Geometry: final body of the model. Coordinates: model frame, mm. A direction names the side the tool comes from. Round coordinates to 2 decimals unless told otherwise and drop trailing zeros. Loops run counter-clockwise (first coordinate to the right, second up) from the corner with the lowest first, then second, coordinate; pieces in that order, holes last. Notation, with made-up numbers: (14, 40) - (24, 40) arc R20 ccw to (24, 76) - close; hole circle Ø3 at (14.5, -38.75). An arc over 180 degrees is marked (long way). Answer in a Markdown table with one row per item. Add a question column.
from build123d import *

# Parameters (mm, degrees)
SKETCH1_R           = 5.5
BOSS_EXTRUDE2_DEPTH = 8.5
SKETCH3_W           = 3.2
SKETCH3_H           = 5.5
CUT_EXTRUDE1_DEPTH  = 6
BOSS_EXTRUDE3_DEPTH = 8.5


with BuildPart() as part:
    # Sketch1 → Boss-Extrude2 (new body)
    with BuildSketch(Plane.XY.offset(20)):
        with Locations((0, 20.92523633)):
            Circle(SKETCH1_R)
    extrude(amount=BOSS_EXTRUDE2_DEPTH)

    # Sketch3 → Cut-Extrude1 (cut)
    with BuildSketch(Plane.XY.offset(28.5)):
        with Locations((0, 20.92523633)):
            Rectangle(SKETCH3_W, SKETCH3_H)
    extrude(amount=-CUT_EXTRUDE1_DEPTH, mode=Mode.SUBTRACT)

    # Sketch4 → Boss-Extrude3 (add)
    with BuildSketch(Plane.XY.offset(20)):
        with BuildLine():
            Line((-0.612805484, 27.420090848), (-0.683508693, 26.382599784))
            ThreePointArc((-0.683508693, 26.382599784), (0, 26.42523633), (0.683508693, 26.382599784))
            Line((0.683508693, 26.382599784), (0.612805484, 27.420090848))
            ThreePointArc((0.612805484, 27.420090848), (0.791416866, 28.376215286), (0.108813843, 29.069128758))
            ThreePointArc((0.108813843, 29.069128758), (0, 29.072382819), (-0.108813843, 29.069128758))
            ThreePointArc((-0.108813843, 29.069128758), (-0.791416866, 28.376215286), (-0.612805484, 27.420090848))
        make_face()
        with BuildLine():
            Line((4.313349752, 25.819485985), (3.760727903, 24.938579779))
            ThreePointArc((3.760727903, 24.938579779), (3.232818888, 25.374829799), (2.654787606, 25.742092438))
            Line((2.654787606, 25.742092438), (3.32180965, 26.539882037))
            ThreePointArc((3.32180965, 26.539882037), (3.739305851, 27.418388093), (4.698827617, 27.577742877))
            ThreePointArc((4.698827617, 27.577742877), (4.788772554, 27.516416295), (4.874892114, 27.449824532))
            ThreePointArc((4.874892114, 27.449824532), (5.01984524, 26.488021768), (4.313349752, 25.819485985))
        make_face()
        with BuildLine():
            Line((6.36634102, 22.349444103), (5.401476877, 21.961598985))
            ThreePointArc((5.401476877, 21.961598985), (5.23081084, 22.624829799), (4.979045272, 23.261709779))
            Line((4.979045272, 23.261709779), (5.987606403, 23.515069401))
            ThreePointArc((5.987606403, 23.515069401), (6.841740827, 23.98039762), (7.711676635, 23.545325605))
            ThreePointArc((7.711676635, 23.545325605), (7.748396757, 23.442843051), (7.778927288, 23.338349376))
            ThreePointArc((7.778927288, 23.338349376), (7.33086335, 22.475033284), (6.36634102, 22.349444103))
        make_face()
        with BuildLine():
            Line((5.987606403, 18.335403259), (4.979045272, 18.588762882))
            ThreePointArc((4.979045272, 18.588762882), (5.23081084, 19.225642861), (5.401476877, 19.888873675))
            Line((5.401476877, 19.888873675), (6.36634102, 19.501028557))
            ThreePointArc((6.36634102, 19.501028557), (7.33086335, 19.375439376), (7.778927288, 18.512123284))
            ThreePointArc((7.778927288, 18.512123284), (7.748396757, 18.407629609), (7.711676635, 18.305147055))
            ThreePointArc((7.711676635, 18.305147055), (6.841740827, 17.87007504), (5.987606403, 18.335403259))
        make_face()
        with BuildLine():
            Line((3.32180965, 15.310590623), (2.654787606, 16.108380222))
            ThreePointArc((2.654787606, 16.108380222), (3.232818888, 16.475642861), (3.760727903, 16.911892881))
            Line((3.760727903, 16.911892881), (4.313349752, 16.030986675))
            ThreePointArc((4.313349752, 16.030986675), (5.01984524, 15.362450892), (4.874892114, 14.400648128))
            ThreePointArc((4.874892114, 14.400648128), (4.788772554, 14.334056365), (4.698827617, 14.272729783))
            ThreePointArc((4.698827617, 14.272729783), (3.739305851, 14.432084567), (3.32180965, 15.310590623))
        make_face()
        with BuildLine():
            Line((-0.612805484, 14.430381812), (-0.683508693, 15.467872876))
            ThreePointArc((-0.683508693, 15.467872876), (0, 15.42523633), (0.683508693, 15.467872876))
            Line((0.683508693, 15.467872876), (0.612805484, 14.430381812))
            ThreePointArc((0.612805484, 14.430381812), (0.791416866, 13.474257374), (0.108813843, 12.781343902))
            ThreePointArc((0.108813843, 12.781343902), (0, 12.778089841), (-0.108813843, 12.781343902))
            ThreePointArc((-0.108813843, 12.781343902), (-0.791416866, 13.474257374), (-0.612805484, 14.430381812))
        make_face()
        with BuildLine():
            Line((-4.313349752, 16.030986675), (-3.760727903, 16.911892881))
            ThreePointArc((-3.760727903, 16.911892881), (-3.232818888, 16.475642861), (-2.654787606, 16.108380222))
            Line((-2.654787606, 16.108380222), (-3.32180965, 15.310590623))
            ThreePointArc((-3.32180965, 15.310590623), (-3.739305851, 14.432084567), (-4.698827617, 14.272729783))
            ThreePointArc((-4.698827617, 14.272729783), (-4.788772554, 14.334056365), (-4.874892114, 14.400648128))
            ThreePointArc((-4.874892114, 14.400648128), (-5.01984524, 15.362450892), (-4.313349752, 16.030986675))
        make_face()
        with BuildLine():
            Line((-6.36634102, 19.501028557), (-5.401476877, 19.888873675))
            ThreePointArc((-5.401476877, 19.888873675), (-5.23081084, 19.225642861), (-4.979045272, 18.588762882))
            Line((-4.979045272, 18.588762882), (-5.987606403, 18.335403259))
            ThreePointArc((-5.987606403, 18.335403259), (-6.841740827, 17.87007504), (-7.711676635, 18.305147055))
            ThreePointArc((-7.711676635, 18.305147055), (-7.748396757, 18.407629609), (-7.778927288, 18.512123284))
            ThreePointArc((-7.778927288, 18.512123284), (-7.33086335, 19.375439376), (-6.36634102, 19.501028557))
        make_face()
        with BuildLine():
            Line((-5.987606403, 23.515069401), (-4.979045272, 23.261709779))
            ThreePointArc((-4.979045272, 23.261709779), (-5.23081084, 22.624829799), (-5.401476877, 21.961598985))
            Line((-5.401476877, 21.961598985), (-6.36634102, 22.349444103))
            ThreePointArc((-6.36634102, 22.349444103), (-7.33086335, 22.475033284), (-7.778927288, 23.338349376))
            ThreePointArc((-7.778927288, 23.338349376), (-7.748396757, 23.442843051), (-7.711676635, 23.545325605))
            ThreePointArc((-7.711676635, 23.545325605), (-6.841740827, 23.98039762), (-5.987606403, 23.515069401))
        make_face()
        with BuildLine():
            Line((-3.32180965, 26.539882037), (-2.654787606, 25.742092438))
            ThreePointArc((-2.654787606, 25.742092438), (-3.232818888, 25.374829799), (-3.760727903, 24.938579779))
            Line((-3.760727903, 24.938579779), (-4.313349752, 25.819485985))
            ThreePointArc((-4.313349752, 25.819485985), (-5.01984524, 26.488021768), (-4.874892114, 27.449824532))
            ThreePointArc((-4.874892114, 27.449824532), (-4.788772554, 27.516416295), (-4.698827617, 27.577742877))
            ThreePointArc((-4.698827617, 27.577742877), (-3.739305851, 27.418388093), (-3.32180965, 26.539882037))
        make_face()
    extrude(amount=BOSS_EXTRUDE3_DEPTH)


solid = part.part
1) Section A-A, the plane x = 5.75. Return the cut outline in (y, z), and give its area (3 significant figures).
2) Reachability of faces 5 (the flat face through (-0.648, 26.909, 24.19)), 6 (the flat face through (1.6, 21, 26)) from +Z, -Z, +X, -X, +Y, -Y: full face, straight path, thin tool, end or side. Return the list, or none.
3) Section C-C, the plane x = -3. Return the cut outline in (y, z).
4) Section B-B, the plane y = 21.5. Return the cut outline in (x, z), and give its area (3 significant figures).
5) Pull-direction query (X, two-part tool) for faces 1 (the flat face through (-2, 21, 28.5)), 2 (the flat face through (4.041, 25.385, 24.19)), 3 (the flat face through (5.49, 18.46, 24.19)), 4 (the cylindrical face through (-5.015, 26.475, 24.19)); classes: pulls with the +X half, pulls with the -X half, needs draft (parallel to the pull), parting line crosses it, or undercut.
6) Contact query for flat-ended pins moving along their axis: pin 1 Ø2 at (y, z) = (26.5, 27.5) entering from -X; pin 2 Ø1 at (x, y) = (-0.5, 21) entering from +Z; pin 3 Ø3 at (x, z) = (5, 25) entering from +Y. Output: stop coordinate, or through.
7) Material intervals for line 1 along X through (y, z) = (15, 25.25); line 2 along X through (y, z) = (23.75, 24.5); line 3 along X through (y, z) = (13.75, 26.5), sorted ascending. Write a range as from..to.
8) Section D-D, the plane y = 17.5. Return the cut outline in (x, z).
Evaluation:
| question | item | result |
|---|---|---|
| 1 | outline | (18.4, 20) - (19.75, 20) - (19.75, 28.5) - (18.4, 28.5) - close; (22.1, 20) - (23.46, 20) - (23.46, 28.5) - (22.1, 28.5) - close |
| 1 | area | 23.0 mm² |
| 2 | face 5 | +Z, -Z |
| 2 | face 6 | +Z |
| 3 | outline | (15.7, 20) - (26.15, 20) - (26.15, 28.5) - (15.7, 28.5) - close |
| 4 | outline | (-5.47, 20) - (5.47, 20) - (5.47, 28.5) - (1.6, 28.5) - (1.6, 22.5) - (-1.6, 22.5) - (-1.6, 28.5) - (-5.47, 28.5) - close |
| 4 | area | 73.8 mm² |
| 5 | face 1 | needs draft |
| 5 | face 2 | pulls with the +X half |
| 5 | face 3 | undercut |
| 5 | face 4 | pulls with the -X half |
| 6 | pin 1 | stops at x = -5.08 |
| 6 | pin 2 | stops at z = 22.5 |
| 6 | pin 3 | stops at y = 27.63 |
| 7 | line 1 | x = -5.08..-3.36, -0.65..0.65, 3.36..5.08 |
| 7 | line 2 | x = -7.52..-6.2, -4.72..4.72, 6.2..7.52 |
| 7 | line 3 | x = -0.84..0.84 |
| 8 | outline | (-4.3, 20) - (4.3, 20) - (4.3, 28.5) - (-4.3, 28.5) - close |
